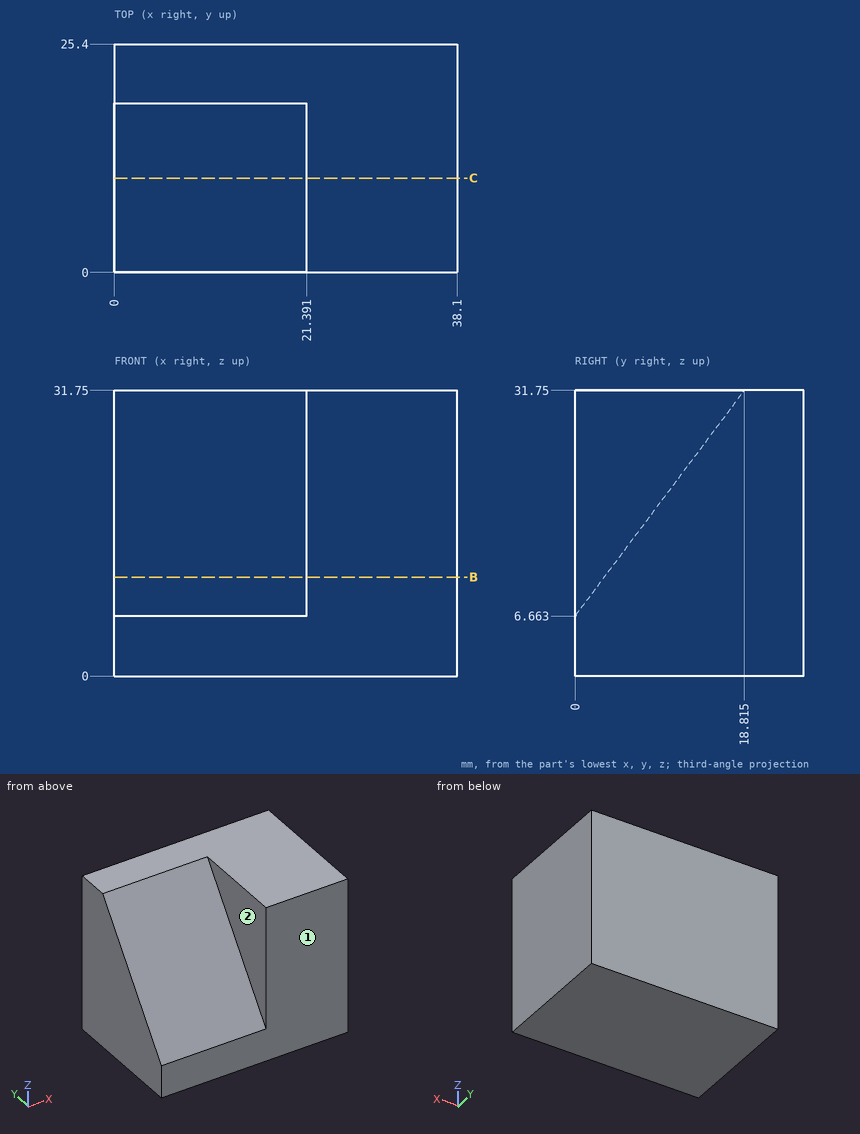
Verification items for this drawing (mm, ordinates from the low corner). A direction names the side the tool comes from. Coordinates: 2 decimals unless noted, no trailing zeros. Write each loop counter-clockwise with the first axis right and the second up, starting at its lowest first coordinate (ties: lowest second). Pieces come first, ordered by that corner, then holes. Notation, with made-up numbers: M 54,54 L 65,54 A33 cw 65,88 Z; hole C -3.5,28.5 d5. An arc over 180 degrees is marked long. Answer as a JSON object with one key per item and string values.
1. Scan lines: L1, parallel to X at y = 2.75, z = 23.5; L2, parallel to Z at x = 16, y = 2.25 (1 decimal); L3, parallel to Z at x = 10, y = 15.75 (1 decimal). Record each from-to range of solid material in increasing order.
Answers below:
{"L1": "x = 21.39 to 38.1", "L2": "z = 0 to 9.7", "L3": "z = 0 to 27.7"}
2. Section check B-B, the plane z = 11. Enter the section's corners in (x, y).
Answers below:
{"outline": "M 0,3.25 L 21.39,3.25 L 21.39,0 L 38.1,0 L 38.1,25.4 L 0,25.4 Z"}
3. Section check C-C, the plane y = 10.5. Enter the section's corners in (x, z).
Answers below:
{"outline": "M 0,0 L 38.1,0 L 38.1,31.75 L 21.39,31.75 L 21.39,20.66 L 0,20.66 Z"}
4. Tool access check on the marked faces 1 and 2. Record the directions out of +Z, -Z, +X, -X, +Y, -Y that give a thin tool (end or side, any length) a straight path to the whole face; none if there is none.
Answers below:
{"face 1": "+Z, -Z, +X, -X, -Y", "face 2": "+Z, -X, -Y"}
5. Go/stop test with a flat-tipped pin: pin 1 Ø10 at (x, z) = (14, 21.5) entering from -Y. Record where the tip stops, or that it passes through.
Answers below:
{"pin 1": "stops at y = 7.38"}
